The figure shows three views and two pictorial views of one solid part (mm, origin at its lowest corner). Answer the questions. A direction names the side the tool comes from. Round coordinates to 2 decimals unless told otherwise and drop trailing zeros. Write each loop counter-clockwise with the first axis right and the second up, starting at its lowest first coordinate (ties: lowest second). Pieces come first, ordered by that corner, then holes.
Item 1: For a pull along X with two mould halves and no side action, classify the marked faces 1, 2, 3 and 4 as +X half, -X half, draft (parallel to the pull), parting line (faces both ways), or undercut.
Item 2: Find section C-C on z = 8.5. Give the vertices of the cut face in (x, y).
Item 3: Find section D-D on y = 7. Give the vertices of the cut face in (x, z).
Item 4: A tool of negligible diameter and unlimited length cuts with its end or side. For the marked faces 5, 6, 7 and 8, from which of +Z, -Z, +X, -X, +Y, -Y can it reach the whole face along a straight path? Write none if from no direction.
Item 5: Each of these flat-tipped pins is pushed along its axis until it touches: pin 1 (1.5 mm diameter, centred on x = 8, y = 17.5, fed in from +Z); pin 2 (1 mm diameter, centred on x = 6.5, z = 5, fed in from -Y); pin 3 (0.8 mm diameter, centred on y = 8, z = 2.5, fed in from -X). Where does it stop, or does it pass through?
Item 6: Find the intervals of material crossed by probe 1 along Y at (x, z) = (6.5, 6.75); probe 2 along Z at (x, y) = (10.25, 3); probe 3 along Z at (x, y) = (12.25, 15.5), in increasing order.
Item 7: Find section B-B on y = 10. Give the vertices of the cut face in (x, z), then the cut area to 3 significant figures.
Item 8: Find section A-A on x = 6.5. Give the vertices of the cut face in (y, z).
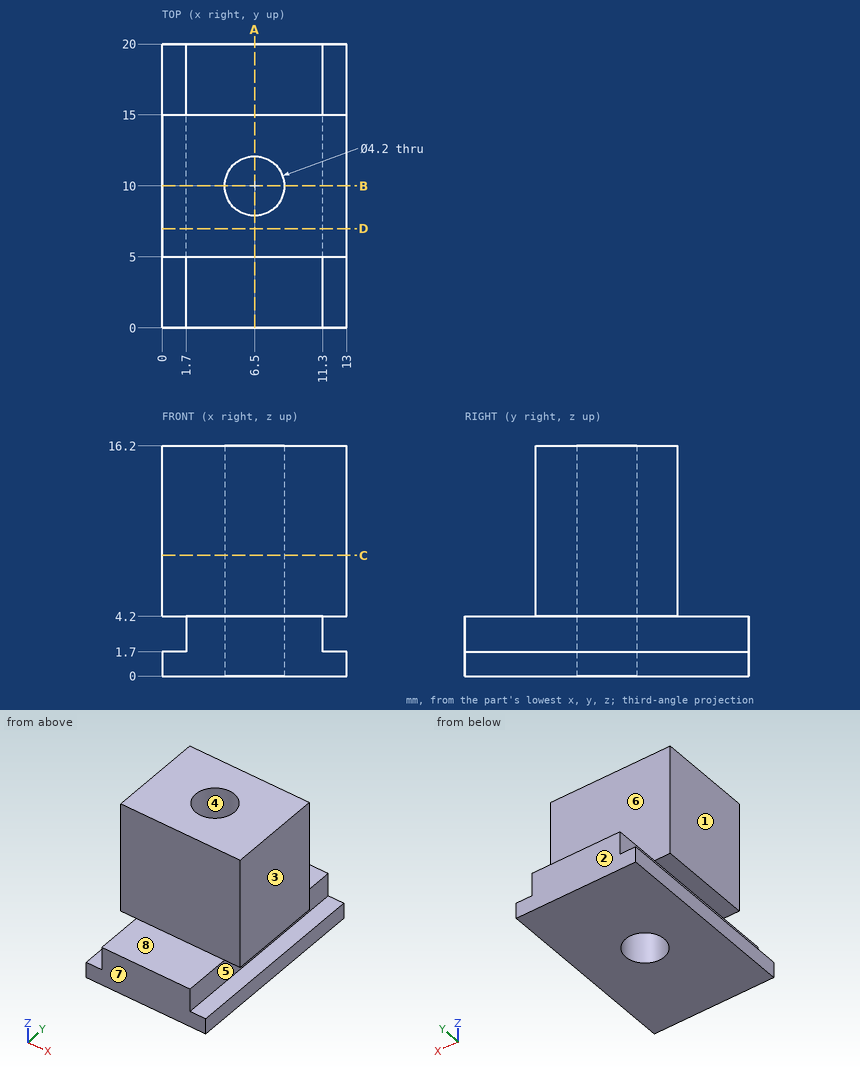
Check values:
1. face 1: -X half
1. face 2: draft
1. face 3: +X half
1. face 4: undercut
2. outline: (0, 5) - (13, 5) - (13, 15) - (0, 15) - close; hole circle Ø4.2 at (6.5, 10)
3. outline: (0, 0) - (13, 0) - (13, 1.7) - (11.3, 1.7) - (11.3, 4.2) - (13, 4.2) - (13, 16.2) - (0, 16.2) - (0, 4.2) - (1.7, 4.2) - (1.7, 1.7) - (0, 1.7) - close
4. face 5: +X, +Y, -Y
4. face 6: +Z, +X, -X, +Y
4. face 7: +Z, -Z, +X, -X, -Y
4. face 8: +Z, +X, -X, -Y
5. pin 1: stops at z = 4.2
5. pin 2: stops at y = 5
5. pin 3: stops at x = 1.7
6. probe 1: y = 5 to 7.9, 12.1 to 15
6. probe 2: z = 0 to 4.2
6. probe 3: z = 0 to 1.7
7. outline: (0, 0) - (4.4, 0) - (4.4, 16.2) - (0, 16.2) - (0, 4.2) - (1.7, 4.2) - (1.7, 1.7) - (0, 1.7) - close; (8.6, 0) - (13, 0) - (13, 1.7) - (11.3, 1.7) - (11.3, 4.2) - (13, 4.2) - (13, 16.2) - (8.6, 16.2) - close
7. area: 134 mm2
8. outline: (0, 0) - (7.9, 0) - (7.9, 16.2) - (5, 16.2) - (5, 4.2) - (0, 4.2) - close; (12.1, 0) - (20, 0) - (20, 4.2) - (15, 4.2) - (15, 16.2) - (12.1, 16.2) - close
